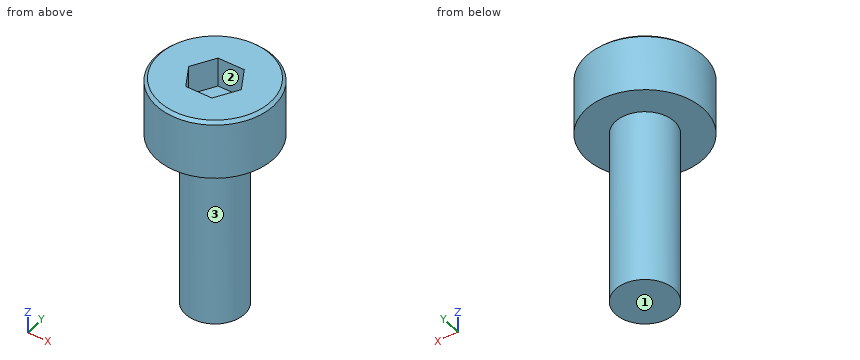
```python
from build123d import *

# Parameters (mm, degrees)
CUT_EXTRUDE_1_DEPTH = 1
CHAMFER_627_SIZE    = 0.1


with BuildPart() as part:
    # 草图1 → 旋转1 (revolve)
    with BuildSketch(Plane(origin=(0, 0, 0), x_dir=(0, 0, -1), z_dir=(1, 0, 0))):
        Polygon((0, 0), (0, 1.99), (2, 1.99), (2, 1), (8, 1), (8, 0), align=None)
    revolve(axis=Axis((0, 0, -8), (0, 0, 1)))

    # 草图2 → 切除-拉伸1 (cut)
    with BuildSketch(Plane.XY):
        Polygon((0.45033321, 0.78), (-0.45033321, 0.78), (-0.90066642, 0), (-0.45033321, -0.78), (0.45033321, -0.78), (0.90066642, 0), align=None)
    extrude(amount=-CUT_EXTRUDE_1_DEPTH, mode=Mode.SUBTRACT)

    # Chamfer 627
    chamfer_627_edges = [part.edges().sort_by_distance(p)[0] for p in [
        (0, -1.99, 0),
    ]]
    chamfer(chamfer_627_edges, length=CHAMFER_627_SIZE)


solid = part.part
```
Source: CAD feature listing. Evaluate the final solid. Frame: model axes, mm. Face numbers are marked on the shaded views. A direction names the side the tool comes from. Round coordinates to 2 decimals unless told otherwise and drop trailing zeros. Loops run counter-clockwise (first coordinate to the right, second up) from the corner with the lowest first, then second, coordinate; pieces in that order, holes last.
1. Contact query for a flat-ended pin moving along its axis: pin 1 (0.8 mm diameter, centred on x = -0.5, y = 0, fed in from +Z). Output: stop coordinate, or through.
2. Section query C-C on z = -4.5. Output: boundary loops of the cut face in (x, y).
3. Access query for the marked faces 1, 2 and 3. Directions: +Z, -Z, +X, -X, +Y, -Y. A direction counts if a zero-diameter tool reaches every point of the face in a straight line with its end or side. Return the directions, or none.
4. Ray query, L1, parallel to Z at x = 1.05, y = -1.55; L2, parallel to Y at x = -0.3, z = -0.75; L3, parallel to Z at x = -0.5, y = -0.55. Return the intervals inside material, ascending.
5. Section query A-A on z = -0.5. Output: boundary loops of the cut face in (x, y).
6. Section query B-B on x = 0. Output: boundary loops of the cut face in (y, z).
Answers below:
1. pin 1: stops at z = 0
2. outline: circle Ø2 at (0, 0)
3. face 1: -Z, +X, -X, +Y, -Y
3. face 2: +Z
3. face 3: -Z
4. L1: z = -2 to 0
4. L2: y = -1.97 to -0.78, 0.78 to 1.97
4. L3: z = -8 to -1
5. outline: circle Ø3.98 at (0, 0); hole (-0.9, 0) - (-0.45, -0.78) - (0.45, -0.78) - (0.9, 0) - (0.45, 0.78) - (-0.45, 0.78) - close
6. outline: (-1.99, -2) - (-1, -2) - (-1, -8) - (1, -8) - (1, -2) - (1.99, -2) - (1.99, -0.1) - (1.89, 0) - (0.78, 0) - (0.78, -1) - (-0.78, -1) - (-0.78, 0) - (-1.89, 0) - (-1.99, -0.1) - close
